Autodesk Inventor part; units mm, degrees
ref_plane "YZ Plane" through (0, 0, 0) normal (1, 0, 0) x (0, 1, 0)
ref_plane "XZ Plane" through (0, 0, 0) normal (0, 1, 0) x (-1, 0, 0)
ref_plane "XY Plane" through (0, 0, 0) normal (0, 0, 1) x (1, 0, 0)
sketch "Sketch1" plane through (0, 0, 0) normal (0, 0, 1) x (1, 0, 0)
  line L0 (0, 0) -> (0, -50.8)
  line L1 (0, -50.8) -> (50.8, -50.8)
  line L2 (3.2258, 0) -> (3.2258, -47.5742)
  line L3 (3.2258, -47.5742) -> (50.8, -47.5742)
  line L4 (0, 0) -> (3.2258, 0)
  line L5 (50.8, -47.5742) -> (50.8, -50.8)
  dimension "d0" = 50.8
  dimension "d1" = 50.8
  dimension "d2" = 3.2258
extrude "Extrusion1" add sketch "Sketch1" along normal blind 1066.8
sketch "Sketch2" plane through (0, -50.8, 0) normal (-1, 0, 0) x (0, 0, 1)
  line L0 (1066.8, 50.8) -> (1066.8, 0)
  line L1 (0, 50.8) -> (0, 0)
  point P0 (160.02, 25.4)
  point P1 (320.04, 25.4)
  point P2 (480.06, 25.4)
  point P3 (640.08, 25.4)
  dimension "d5" = 1066.8
hole "Hole1" at (0, -25.4, 480.06) at (0, -25.4, 640.08) at (0, -25.4, 320.04) at (0, -25.4, 160.02) direction (1, 0, 0) diameter 14.605 end through all
sketch "Sketch3" plane through (0, -50.8, 0) normal (-1, 0, 0) x (0, 0, 1)
  point P0 (0, 50.8)
  point P1 (797.56, 25.4)
  point P2 (957.58, 25.4)
properties part number "angle al 1.5x1.5 (48)"
Verification items for the finished model (mm, model axes). A direction names the side the tool comes from. Coordinates: 2 decimals unless noted, no trailing zeros. Write each loop counter-clockwise with the first axis right and the second up, starting at its lowest first coordinate (ties: lowest second). Pieces come first, ordered by that corner, then holes. Notation, with made-up numbers: M 24.25,-10 L 56.25,-10 A26 cw 56.25,25 Z; hole C 5.5,-1.75 d8. An arc over 180 degrees is marked long. Use CSV: the item, a comma, the result in double quotes.
Q1. Set-up check for faces 1 (the flat face through (3, -37, 0)), 2 (the flat face through (3.226, -23, 526)): record each of +Z, -Z, +X, -X, +Y, -Y from which the full face is reachable in a straight line by a thin tool's end or side.
Computed values:
face 1,"-Z, +X, -X, +Y, -Y"
face 2,"+Z, -Z, +X, +Y"
Q2. Thickness scan on line 1 along Z through (x, y) = (1.2, -25.4); line 2 along Y through (x, z) = (0.75, 160.02); line 3 along Y through (x, z) = (29, 199.5). Record the ranges inside material, lowest first. Write a range as [from, to].
Computed values:
line 1,"[0, 152.72], [167.32, 312.74], [327.34, 472.76], [487.36, 632.78], [647.38, 1066.8]"
line 2,"[-50.8, -32.7], [-18.1, 0]"
line 3,"[-50.8, -47.57]"
Q3. Go/stop test with flat-tipped pins: P1, Ø14.5, axis at y = -24.5, z = 743, coming from the +X side; P2, Ø10, axis at x = 40.5, z = 214.5, coming from the +Y side. Record where each tip stops, or that it passes through.
Computed values:
P1,"x = 3.23"
P2,"y = -47.57"
Q4. Section check A-A, the plane z = 76. Enter the section's corners in (x, y).
Computed values:
outline,"M 0,-50.8 L 50.8,-50.8 L 50.8,-47.57 L 3.23,-47.57 L 3.23,0 L 0,0 Z"
Q5. Section check B-B, the plane x = 43. Enter the section's corners in (y, z).
Computed values:
outline,"M -50.8,0 L -47.57,0 L -47.57,1066.8 L -50.8,1066.8 Z"
Q6. Mould release check, pull along Y, two halves, no side actions. Record for faces 3 (the flat face through (27, -47.574, 526)), 4 (the flat face through (25, -50.8, 526)), 5 (the flat face through (0, -25, 526)): pulls with the +Y half, pulls with the -Y half, needs draft (parallel to the pull), parting line crosses it, or undercut.
Computed values:
face 3,"pulls with the +Y half"
face 4,"pulls with the -Y half"
face 5,"needs draft"
